Can you work these out from the model? Positions are in its coordinate system, mm. Face numbers are marked on the shaded views. A direction names the side the tool comes from. Coordinates: 2 decimals unless noted, no trailing zeros. Order: outer loops, then holes, each group sorted by start corner. A loop starts at its lowest first (then second) coordinate and runs counter-clockwise, first axis right, second up. Notation, with made-up numbers: M 5,72.25 L 14,72.25 A16 cw 14,90.25 Z; hole C -7.5,24 d6. An arc over 180 degrees is marked long. Answer as a JSON object with one key per item and string values.
from build123d import *

# Parameters (mm, degrees)
F1_DEPTH = 25.4
F2_W     = 12.9091180861
F2_H     = 25.0910650939
F3_DEPTH = 28.702


with BuildPart() as f1:
    # F0 (on Front) → F1 (new body)
    with BuildSketch(Plane.XZ):
        with BuildLine():
            Line((-33.6216918521, 56.1617612839), (-53.54340747, 56.1617612839))
            Line((-53.54340747, 56.1617612839), (-53.54340747, 38.7188270688))
            Line((-53.54340747, 38.7188270688), (-21.719571203, 38.7188270688))
            Line((-21.719571203, 38.7188270688), (-21.719571203, 54.4453912809))
            ThreePointArc((-21.719571203, 54.4453912809), (-28.4139375356, 50.1491411825), (-33.6216918521, 56.1617612839))
        make_face()
        with BuildLine():
            ThreePointArc((-21.4720585056, 56.1617612839), (-27.5468751788, 62.2365779571), (-33.6216918521, 56.1617612839))
            Line((-33.6216918521, 56.1617612839), (-21.719571203, 56.1617612839))
            Line((-21.719571203, 56.1617612839), (-21.719571203, 54.4453912809))
            ThreePointArc((-21.719571203, 54.4453912809), (-21.5342550775, 55.2946989271), (-21.4720585056, 56.1617612839))
        make_face()
        with BuildLine():
            Line((-21.719571203, 56.1617612839), (-33.6216918521, 56.1617612839))
            ThreePointArc((-33.6216918521, 56.1617612839), (-28.4139375356, 50.1491411825), (-21.719571203, 54.4453912809))
            Line((-21.719571203, 54.4453912809), (-21.719571203, 56.1617612839))
        make_face()
    extrude(amount=F1_DEPTH)

    # F2 (on Front) → F3 (cut)
    with BuildSketch(Plane.XZ):
        with Locations((-42.769966647, 38.8393672183)):
            Rectangle(F2_W, F2_H)
    extrude(amount=F3_DEPTH, mode=Mode.SUBTRACT)


solid = f1.part
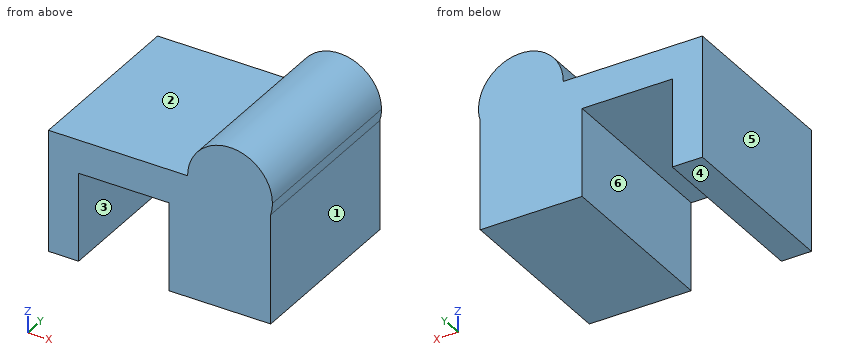
Item 1: Please list where these lines run through material, in increasing order: line 1 (X direction, y = -12.75, z = 46.25); line 2 (Z direction, x = -50, y = -19.25); line 3 (Z direction, x = -46.5, y = -23.5).
Answers follow:
{"line 1": "x = -53.54 to -49.22, -36.32 to -21.72", "line 2": "z = 38.72 to 56.16", "line 3": "z = 51.38 to 56.16"}
Item 2: I want a section at A-A, the plane z = 43.25. Write out the boundary of the cut face in (x, y).
Answers follow:
{"outline": "M -53.54,-25.4 L -49.22,-25.4 L -49.22,0 L -53.54,0 Z; M -36.32,-25.4 L -21.72,-25.4 L -21.72,0 L -36.32,0 Z"}
Item 3: I want a section at D-D, the plane z = 58. Write out the boundary of the cut face in (x, y), plus the area to 3 significant figures.
Answers follow:
{"outline": "M -33.34,-25.4 L -21.76,-25.4 L -21.76,0 L -33.34,0 Z", "area": "294 mm^2"}
Item 4: I want a section at C-C, the plane x = -41.5. Write out the boundary of the cut face in (y, z), plus the area to 3 significant figures.
Answers follow:
{"outline": "M -25.4,51.38 L 0,51.38 L 0,56.16 L -25.4,56.16 Z", "area": "121 mm^2"}
Item 5: I'm going to push flat-ended pins straight in: pin 1 (4 mm diameter, centred on y = -10, z = 46.5, fed in from +X); pin 2 (10 mm diameter, centred on x = -43.5, y = -12, fed in from +Z); pin 3 (4 mm diameter, centred on x = -43, y = -17.5, fed in from -Z). Where does each tip first touch, or does it pass through?
Answers follow:
{"pin 1": "stops at x = -21.72", "pin 2": "stops at z = 56.16", "pin 3": "stops at z = 51.38"}
Item 6: Which directions (+Z, -Z, +X, -X, +Y, -Y) give clear straight access to the entire face, cutting with the end or side of a thin tool? Please do the marked faces 1, 2 and 3.
Answers follow:
{"face 1": "-Z, +X, +Y, -Y", "face 2": "+Z, -X, +Y, -Y", "face 3": "-Z, +Y, -Y"}
Item 7: If we mould it in two halves opening along X, with no side actions, what happens to the marked faces 4, 5 and 6? For each: pulls with the +X half, pulls with the -X half, needs draft (parallel to the pull), parting line crosses it, or undercut.
Answers follow:
{"face 4": "needs draft", "face 5": "pulls with the -X half", "face 6": "undercut"}
Item 8: I want a section at B-B, the plane y = -20.75. Write out the boundary of the cut face in (x, z), plus the area to 3 significant figures.
Answers follow:
{"outline": "M -53.54,38.72 L -49.22,38.72 L -49.22,51.38 L -36.32,51.38 L -36.32,38.72 L -21.72,38.72 L -21.72,54.45 A6.07 ccw long -33.62,56.16 L -53.54,56.16 Z", "area": "450 mm^2"}
